from build123d import *

# Parameters (mm, degrees)
SKETCH1_R           = 4
BOSS_EXTRUDE1_DEPTH = 3


with BuildPart() as part:
    # Sketch1 → Boss-Extrude1 (new body)
    with BuildSketch(Plane.XY):
        with BuildLine():
            Line((104.119192453, 179.407061364), (134.119192453, 179.874374377))
            Line((134.119192453, 179.874374377), (134.119192453, 165.874374377))
            Line((134.119192453, 165.874374377), (131.119192453, 165.874374377))
            Line((131.119192453, 165.874374377), (131.119192453, 157.874374377))
            Line((131.119192453, 157.874374377), (134.119192453, 157.874374377))
            Line((134.119192453, 157.874374377), (134.119192453, 153.374336284))
            Line((134.119192453, 153.374336284), (123.963204023, 153.374336284))
            Line((123.963204023, 153.374336284), (123.963204023, 148.374336284))
            Line((123.963204023, 148.374336284), (134.119192453, 148.374336284))
            Line((134.119192453, 148.374336284), (134.119192453, 143.874374377))
            Line((134.119192453, 143.874374377), (131.119192453, 143.874374377))
            Line((131.119192453, 143.874374377), (131.119192453, 135.874374377))
            Line((131.119192453, 135.874374377), (134.119192453, 135.874374377))
            Line((134.119192453, 135.874374377), (134.119192453, 121.874374377))
            Line((134.119192453, 121.874374377), (104.119206498, 121.903403691))
            ThreePointArc((104.119206498, 121.903403691), (97.58987401, 125.424418251), (93.963204023, 131.895661647))
            Line((93.963204023, 131.895661647), (93.963204023, 169.853170932))
            ThreePointArc((93.963204023, 169.853170932), (97.844114816, 175.902641249), (104.119192453, 179.407061364))
        make_face()
        with Locations((113.963204023, 150.874376287)):
            Circle(SKETCH1_R, mode=Mode.SUBTRACT)
    extrude(amount=BOSS_EXTRUDE1_DEPTH)


solid = part.part
Could you check a few things on this model? Use its own coordinates, in mm. A direction names the side the tool comes from. Coordinates: 2 decimals unless noted, no trailing zeros. Loops run counter-clockwise (first coordinate to the right, second up) from the corner with the lowest first, then second, coordinate; pieces in that order, holes last.
1. For P1, Ø1, axis at x = 106.5, z = 1.5, coming from the -Y side; P2, Ø1, axis at x = 102, z = 2.5, coming from the +Y side; P3, Ø7, axis at x = 113.96, y = 150.87, coming from the +Z side; P4, Ø0.9, axis at y = 141.5, z = 1, coming from the +X side, each with a flat end and sliding along its axis, tell me the tip position at first contact or that it passes through.
2. Imagine slicing it at C-C (y = 164). Please give me the cut outline in (x, z).
3. I need wall thicknesses on L1, parallel to Y at x = 132.5, z = 0.9; L2, parallel to Y at x = 105, z = 1; L3, parallel to Y at x = 117, z = 0.5. Which ranges of each line are inside material? Lowest first, please.
4. Imagine slicing it at B-B (z = 2.4). Please give me the cut outline in (x, y) (3 decimals), and give its area (3 significant figures).
5. For faces 1 (the face through (133, 135.874, 1)), 2 (the face through (134.119, 129, 1)), which set-ups out of +Z, -Z, +X, -X, +Y, -Y let a thin tool reach every point of the face, with its end or its side?
6. Imagine slicing it at A-A (x = 128). Please give me the cut outline in (y, z), and give its area (3 significant figures).
7. We'd pull the mould along X, two halves only. Please class faces 3 (the face through (97.665, 125.351, 1.479)), 4 (the face through (119, 151, 0)), 5 (the face through (111.015, 153.578, 1.479)), 6 (the face through (134.119, 173, 1)): released by +X, released by -X, zero draft, split by the parting line, or undercut.
Computed values:
1. P1: stops at y = 121.9
1. P2: stops at y = 178.87
1. P3: passes through
1. P4: stops at x = 131.12
2. outline: (93.96, 0) - (131.12, 0) - (131.12, 3) - (93.96, 3) - close
3. L1: y = 121.88 to 135.87, 143.87 to 148.37, 153.37 to 157.87, 165.87 to 179.85
3. L2: y = 121.9 to 179.42
3. L3: y = 121.89 to 148.27, 153.48 to 179.61
4. outline: (93.963, 131.896) arc R13.296 ccw to (104.119, 121.903) - (134.119, 121.874) - (134.119, 135.874) - (131.119, 135.874) - (131.119, 143.874) - (134.119, 143.874) - (134.119, 148.374) - (123.963, 148.374) - (123.963, 153.374) - (134.119, 153.374) - (134.119, 157.874) - (131.119, 157.874) - (131.119, 165.874) - (134.119, 165.874) - (134.119, 179.874) - (104.119, 179.407) arc R14.784 ccw to (93.963, 169.853) - close; hole circle Ø8 at (113.963, 150.874)
4. area: 2,100 mm2
5. face 1: +Z, -Z, +X
5. face 2: +Z, -Z, +X, +Y, -Y
6. outline: (121.88, 0) - (148.37, 0) - (148.37, 3) - (121.88, 3) - close; (153.37, 0) - (179.78, 0) - (179.78, 3) - (153.37, 3) - close
6. area: 159 mm2
7. face 3: released by -X
7. face 4: zero draft
7. face 5: undercut
7. face 6: released by +X
